The listing builds one solid part. Answer for the finished solid, in the listing's coordinates (mm). Face numbers are marked on the shaded views. Round coordinates to 2 decimals unless told otherwise and drop trailing zeros. Order: outer loops, then holes, each group sorted by start corner. A loop starts at its lowest first (then second) coordinate and runs counter-clockwise, first axis right, second up. Notation, with made-up numbers: M 1,56 L 8,56 A25 cw 8,71 Z; hole C -26,85 d2. An arc over 180 degrees is marked long. Write item = value, one per line. Start each with the question number.
(1) A cutting plane is placed at A-A, the plane y = 61. Determine the outline of the cut face in (x, z).
(2) Straight lines are drawn through the part: probe 1 along Z at (x, y) = (-14.5, 28); probe 2 along Y at (x, z) = (0, -28.2); probe 3 along Y at (x, z) = (28.7, 0). For each, find the intervals that lie inside material, in ascending order. Write a range as from..to.
(3) For a pull along Z with two mould halves and no side action, classify the marked faces 1, 2 and 3 as released by +Z, released by -Z, zero draft, split by the parting line, or undercut.
(4) Each of these flat-tipped pins is pushed along its axis until it touches: pin 1 (7.5 mm diameter, centred on y = 33, z = 1.5, fed in from +X); pin 2 (7.5 mm diameter, centred on y = 30.5, z = -2.5, fed in from -X); pin 3 (6 mm diameter, centred on x = -18.5, y = 9, fed in from -Z). Where does it stop, or does it pass through?
(5) A cutting plane is placed at B-B, the plane y = -30. Determine the outline of the cut face in (x, z).
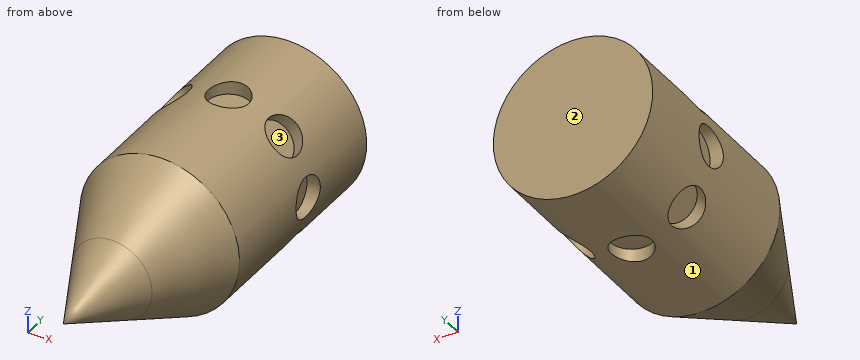
from build123d import *

# Parameters (mm, degrees)
SKETCH2_R          = 7.615394345
CUT_EXTRUDE1_DEPTH = 5
CIRPATTERN1_COUNT  = 8


with BuildPart() as part:
    # Sketch1 → Revolve1 (revolve)
    with BuildSketch(Plane.XY, mode=Mode.PRIVATE) as revolve1_sk:
        Polygon((-29.836570739, 70.106190724), (0, 70.106190724), (0, -39.684589186), (0, -70.111322573), (-15.015790503, -39.684589186), (-29.836570739, -9.65300818), align=None)
    revolve(revolve1_sk.sketch.rotate(Axis((0, 70.106190724, 0), (0, -1, 0)), 270), axis=Axis((0, 70.106190724, 0), (0, -1, 0)))

    # Sketch2 → Cut-Extrude1 (cut)
    with BuildSketch(Plane.XY.offset(29.836570739)):
        with Locations((0, 33.406581413)):
            Circle(SKETCH2_R)
    cut_extrude1 = extrude(amount=-CUT_EXTRUDE1_DEPTH, mode=Mode.SUBTRACT)

    # CirPattern1: Cut-Extrude1 ×8 about axis
    cirpattern1_axis = Axis((0, 0, 0), (0, 1, 0))
    for i in range(1, CIRPATTERN1_COUNT):
        add(cut_extrude1.rotate(cirpattern1_axis, i * 360 / CIRPATTERN1_COUNT), mode=Mode.SUBTRACT)


solid = part.part
Reported:
q1.outline = C 0,0 d59.67
q2.probe_1 = -26.08..-22.08, -20.62..20.62, 22.08..26.08
q2.probe_2 = -12.97..25.79, 41.02..70.11
q2.probe_3 = -11.96..25.79, 41.02..70.11
q3.face_1 = split by the parting line
q3.face_2 = zero draft
q3.face_3 = undercut
q4.pin_1 = 24.84
q4.pin_2 = -24.84
q4.pin_3 = -25.49
q5.outline = C 0,0 d39.59
